Autodesk Inventor part; units mm, degrees
ref_plane "YZ Plane" through (0, 0, 0) normal (1, 0, 0) x (0, 1, 0)
ref_plane "XZ Plane" through (0, 0, 0) normal (0, 1, 0) x (-1, 0, 0)
ref_plane "XY Plane" through (0, 0, 0) normal (0, 0, 1) x (1, 0, 0)
sketch "Sketch1" plane through (0, 0, 0) normal (0, 0, 1) x (1, 0, 0)
  line L0 (0, 0) -> (1, 0)
  line L1 (1, 0) -> (1, 1.95)
  line L2 (1, 1.95) -> (0, 1.95)
  line L3 (0, 1.95) -> (0, 0)
  line L4 (1, 0) -> (2.7, 0)
  line L5 (2.7, 0) -> (2.7, 2.5)
  line L6 (2.7, 2.5) -> (1, 2.5)
  line L7 (1, 2.5) -> (1, 0)
  line L8 (2.7, 0) -> (3.9, 0)
  line L9 (3.9, 0) -> (3.9, 1.85)
  line L10 (3.9, 1.85) -> (2.7, 1.85)
  line L11 (2.7, 1.85) -> (2.7, 0)
  line L12 (3.9, 0) -> (5.1, 0)
  line L13 (5.1, 0) -> (5.1, 2)
  line L14 (5.1, 2) -> (3.9, 2)
  line L15 (3.9, 2) -> (3.9, 0)
  line L16 (5.1, 0) -> (7.4, 0)
  line L17 (7.4, 0) -> (7.4, 4)
  line L18 (7.4, 4) -> (5.1, 4)
  line L19 (5.1, 4) -> (5.1, 0)
  line L20 (7.4, 0) -> (8.6, 0)
  line L21 (8.6, 0) -> (8.6, 2)
  line L22 (8.6, 2) -> (7.4, 2)
  line L23 (7.4, 2) -> (7.4, 0)
  line L24 (8.6, 0) -> (9.5, 0)
  line L25 (9.5, 0) -> (9.5, 4)
  line L26 (9.5, 4) -> (8.6, 4)
  line L27 (8.6, 4) -> (8.6, 0)
  line L28 (9.5, 0) -> (11, 0)
  line L29 (11, 0) -> (11, 2)
  line L30 (11, 2) -> (9.5, 2)
  line L31 (9.5, 2) -> (9.5, 0)
  line L32 (11, 0) -> (13.5, 0)
  line L33 (13.5, 0) -> (13.5, 1.375)
  line L34 (13.5, 1.375) -> (11, 1.375)
  line L35 (11, 1.375) -> (11, 0)
  dimension "d0" = 2.75
  dimension "d1" = 13.5
  dimension "d2" = 4
  dimension "d3" = 3.7
  dimension "d4" = 3.9
  dimension "d5" = 8
  dimension "d6" = 4
  dimension "d7" = 1
  dimension "d8" = 2.7
  dimension "d9" = 11
  dimension "d10" = 9.5
  dimension "d11" = 8.6
  dimension "d12" = 7.4
  dimension "d13" = 5.1
  dimension "d14" = 3.9
  dimension "d25" = 5
revolve "Revolution1" add sketch "Sketch1" angle 360 about axis through (0, 0, 0) along (1, 0, 0)
hole "Hole1" at (0, 0, 0) direction (1, 0, 0) diameter 1.567 depth 6.5 tip angle 118 counterbore diameter 2 counterbore depth 2
properties part number "403-10" material "Brass, Soft Yellow"
Geometry check sheet. Reference: the model listing, model coordinates, mm. A direction names the side the tool comes from. Give positions to 0.01 mm unless a question says otherwise; leave off trailing zeros. Write each loop counter-clockwise with the first axis right and the second up, starting at its lowest first coordinate (ties: lowest second). Pieces come first, ordered by that corner, then holes. Notation, with made-up numbers: (72, -25.75) - (79, -25.75) arc R19 cw to (79, -20.75) - close; hole circle Ø10 at (76, -18). An arc over 180 degrees is marked (long way). Put each result on its own line as item: value.
1. Set-up check for faces 4 (the flat face through (0, 1, -1)), 5 (the cylindrical face through (4.492, -0.434, 1.952)), 6 (the cylindrical face through (12.23, -0.3, 1.34)), 7 (the cylindrical face through (1, 1, 0)): record each of +Z, -Z, +X, -X, +Y, -Y from which the full face is reachable in a straight line by a thin tool's end or side.
Ans:
face 4: +Z, -Z, -X, +Y, -Y
face 5: none
face 6: +X
face 7: -X
2. Go/stop test with flat-tipped pins: pin 1 (1.8 mm diameter, centred on y = 0, z = 0, fed in from -X); pin 2 (1.5 mm diameter, centred on x = 9, z = -3, fed in from -Y); pin 3 (1.5 mm diameter, centred on y = 3, z = -1.5, fed in from -X). Record where each tip stops, or that it passes through.
Ans:
pin 1: stops at x = 2
pin 2: stops at y = -3.31
pin 3: stops at x = 5.1
3. Sectioned sample at D-D, the plane x = 5.5. Enter the section's corners in (y, z), plus the area to 3 significant figures.
Ans:
outline: circle Ø8 at (0, 0); hole circle Ø1.57 at (0, 0)
area: 48.3 mm²
4. Draft check along Y on faces 1 (the flat face through (8.6, -2, -1)), 2 (the cylindrical face through (1.84, -0.54, 2.44)), 3 (the cylindrical face through (4.281, -0.235, 0.747)). Enter one of: +Y half, -Y half, draft (parallel to the pull), parting line (faces both ways), or undercut.
Ans:
face 1: draft
face 2: parting line
face 3: undercut
5. Sectioned sample at A-A, the plane z = 3. Enter the section's corners in (x, y), plus the area to 3 significant figures.
Ans:
outline: (5.1, -2.65) - (7.4, -2.65) - (7.4, 2.65) - (5.1, 2.65) - close; (8.6, -2.65) - (9.5, -2.65) - (9.5, 2.65) - (8.6, 2.65) - close
area: 16.9 mm²
6. Sectioned sample at C-C, the plane x = 3. Enter the section's corners in (y, z), plus the area to 3 significant figures.
Ans:
outline: circle Ø3.7 at (0, 0); hole circle Ø1.57 at (0, 0)
area: 8.82 mm²
7. Thickness scan on line 1 (X direction, y = 1, z = 2.25); line 2 (X direction, y = 0, z = 3); line 3 (Z direction, x = 4.55, y = 0). Record the ranges inside material, lowest first.
Ans:
line 1: x = 1 to 2.7, 5.1 to 7.4, 8.6 to 9.5
line 2: x = 5.1 to 7.4, 8.6 to 9.5
line 3: z = -2 to -0.78, 0.78 to 2
